from build123d import *

# Parameters (mm, degrees)
F1_DEPTH = 3.175


with BuildPart() as f1:
    # F0 (on Top) → F1 (new body)
    with BuildSketch(Plane.XY):
        Polygon((120, 75), (120, 80), (115, 80), (115, 83.175), (105, 83.175), (105, 80), (95, 80), (95, 83.175), (85, 83.175), (85, 80), (75, 80), (75, 83.175), (65, 83.175), (65, 80), (55, 80), (55, 83.175), (45, 83.175), (45, 80), (35, 80), (35, 83.175), (25, 83.175), (25, 80), (15, 80), (15, 83.175), (5, 83.175), (5, 80), (0, 80), (-5, 80), (-5, 83.175), (-15, 83.175), (-15, 80), (-25, 80), (-25, 83.175), (-35, 83.175), (-35, 80), (-45, 80), (-45, 83.175), (-55, 83.175), (-55, 80), (-65, 80), (-65, 83.175), (-75, 83.175), (-75, 80), (-85, 80), (-85, 83.175), (-95, 83.175), (-95, 80), (-105, 80), (-105, 83.175), (-115, 83.175), (-115, 80), (-120, 80), (-120, 75), (-123.175, 75), (-123.175, 65), (-120, 65), (-120, 55), (-123.175, 55), (-123.175, 45), (-120, 45), (-120, 35), (-123.175, 35), (-123.175, 25), (-120, 25), (-120, 15), (-123.175, 15), (-123.175, 5), (-120, 5), (-120, 0), (-120, -5), (-123.175, -5), (-123.175, -15), (-120, -15), (-120, -25), (-123.175, -25), (-123.175, -35), (-120, -35), (-120, -45), (-123.175, -45), (-123.175, -55), (-120, -55), (-120, -65), (-123.175, -65), (-123.175, -75), (-120, -75), (-120, -80), (-115, -80), (-115, -83.175), (-105, -83.175), (-105, -80), (-95, -80), (-95, -83.175), (-85, -83.175), (-85, -80), (-75, -80), (-75, -83.175), (-65, -83.175), (-65, -80), (-55, -80), (-55, -83.175), (-45, -83.175), (-45, -80), (-35, -80), (-35, -83.175), (-25, -83.175), (-25, -80), (-15, -80), (-15, -83.175), (-5, -83.175), (-5, -80), (0, -80), (5, -80), (5, -83.175), (15, -83.175), (15, -80), (25, -80), (25, -83.175), (35, -83.175), (35, -80), (45, -80), (45, -83.175), (55, -83.175), (55, -80), (65, -80), (65, -83.175), (75, -83.175), (75, -80), (85, -80), (85, -83.175), (95, -83.175), (95, -80), (105, -80), (105, -83.175), (115, -83.175), (115, -80), (120, -80), (120, -75), (123.175, -75), (123.175, -65), (120, -65), (120, -55), (123.175, -55), (123.175, -45), (120, -45), (120, -35), (123.175, -35), (123.175, -25), (120, -25), (120, -15), (123.175, -15), (123.175, -5), (120, -5), (120, 0), (120, 5), (123.175, 5), (123.175, 15), (120, 15), (120, 25), (123.175, 25), (123.175, 35), (120, 35), (120, 45), (123.175, 45), (123.175, 55), (120, 55), (120, 65), (123.175, 65), (123.175, 75), align=None)
    extrude(amount=F1_DEPTH)


solid = f1.part
Geometry check sheet. Reference: the model listing, model coordinates, mm. Coordinates: 2 decimals unless noted, no trailing zeros. Order: outer loops, then holes, each group sorted by start corner. A loop starts at its lowest first (then second) coordinate and runs counter-clockwise, first axis right, second up. Notation, with made-up numbers: (37, 67) - (53, 67) arc R13 cw to (53, 73) - close; hole circle Ø6 at (70.5, 74). An arc over 180 degrees is marked (long way). Answer in a Markdown table with one row per item. Add a question column.
1) Cross-section at A-A, the plane y = 60. Record the cut outline in (x, z) (3 decimals), then the cut area to 3 significant figures.
2) Material ranges on line 1 along X through (y, z) = (-60, 1.95); line 2 along Y through (x, z) = (80, 2.85), recorded low to high. Write a range as [from, to].
3) Gauge pin test, flat ends, axial feed: P1, Ø1, axis at x = -58.5, z = 2.5, coming from the -Y side; P2, Ø1.5, axis at y = -63, z = 1, coming from the +X side; P3, Ø1.6, axis at x = -122, z = 1.5, coming from the -Y side. Record the tip position at first contact, or that the pin passes through.
4) Cross-section at B-B, the plane x = -99. Record the cut outline in (y, z) (3 decimals), then the cut area to 3 significant figures.
Check result:
| question | item | result |
|---|---|---|
| 1 | outline | (-120, 0) - (120, 0) - (120, 3.175) - (-120, 3.175) - close |
| 1 | area | 762 mm² |
| 2 | line 1 | x = [-120, 120] |
| 2 | line 2 | y = [-80, 80] |
| 3 | P1 | stops at y = -80 |
| 3 | P2 | stops at x = 120 |
| 3 | P3 | stops at y = -75 |
| 4 | outline | (-80, 0) - (80, 0) - (80, 3.175) - (-80, 3.175) - close |
| 4 | area | 508 mm² |
